Could you check a few things on this drawing? It's one solid part, dimensions in mm from its lowest x, y, z. Give positions to 0.01 mm unless a question says otherwise; leave off trailing zeros. Loops run counter-clockwise (first coordinate to the right, second up) from the corner with the lowest first, then second, coordinate; pieces in that order, holes last. Notation, with made-up numbers: (-39, -30) -> (-32, -30) arc R14 cw to (-32, -25) -> close; hole circle Ø8 at (87, 6). An arc over 180 degrees is marked (long way). Use CSV: the item, a comma, the result in double quotes.
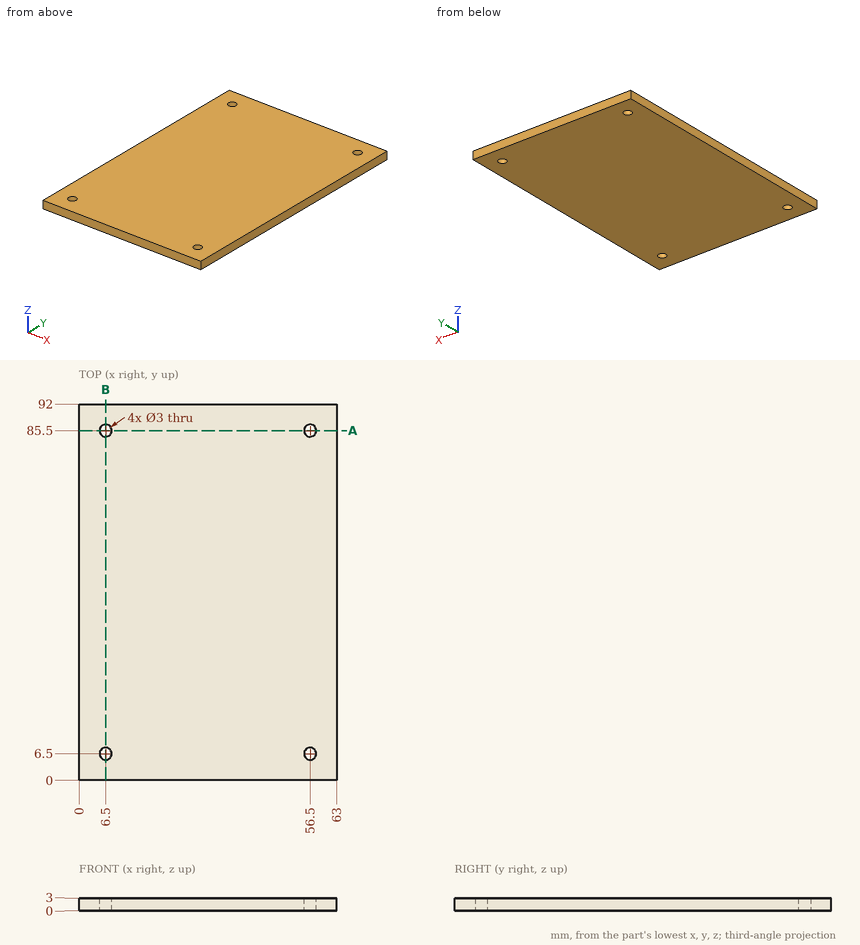
(1) If we section it at A-A, the plane y = 85.5: Write out the boundary of the cut face in (x, z).
Answer sheet:
outline,"(0, 0) -> (5, 0) -> (5, 3) -> (0, 3) -> close; (8, 0) -> (55, 0) -> (55, 3) -> (8, 3) -> close; (58, 0) -> (63, 0) -> (63, 3) -> (58, 3) -> close"
(2) Will this pin go through, and if not, where does the flat tip stop? pin 1 Ø2.5 at (x, y) = (56.5, 85.5) entering from -Z.
Answer sheet:
pin 1,"passes through"
(3) If I drill on L1, parallel to X at y = 85.5, z = 1.8; L2, parallel to Y at x = 56.5, z = 0.9; L3, parallel to Y at x = 56, z = 2.85, over which ranges is the centre line in solid material (lowest first)? Write a range as from..to.
Answer sheet:
L1,"x = 0..5, 8..55, 58..63"
L2,"y = 0..5, 8..84, 87..92"
L3,"y = 0..5.09, 7.91..84.09, 86.91..92"
(4) If we section it at B-B, the plane x = 6.5: Write out the boundary of the cut face in (y, z), then the cut area to 3 significant figures.
Answer sheet:
outline,"(0, 0) -> (5, 0) -> (5, 3) -> (0, 3) -> close; (8, 0) -> (84, 0) -> (84, 3) -> (8, 3) -> close; (87, 0) -> (92, 0) -> (92, 3) -> (87, 3) -> close"
area,"258 mm2"
